Can you work these out from the model? Positions are in its coordinate system, mm. A direction names the side the tool comes from. Round coordinates to 2 decimals unless told otherwise and drop trailing zeros. Loops run counter-clockwise (first coordinate to the right, second up) from the corner with the lowest first, then second, coordinate; pieces in that order, holes last.
(1) Which directions (+Z, -Z, +X, -X, +Y, -Y) give clear straight access to the entire face, cutting with the end or side of a thin tool? Please do faces 1 (the face through (-228.3, -4, 45)), 2 (the face through (-3, -6, 88)), 3 (the face through (228.3, -4, 45)).
(2) I want a section at A-A on y = -3. Write out the boundary of the cut face in (x, z), plus the area to 3 significant figures.
(3) If I drill on line 1 along Z through (x, y) = (-195.5, -5.75); line 2 along X through (y, z) = (-2.5, 55); line 3 along Y through (x, z) = (-77.5, 7), over which ranges is the centre line in solid material (lowest first)?
(4) Will these pins go through, and if not, where does the flat tip stop? pin 1 Ø1.2 at (x, z) = (-230, 41) entering from +Y; pin 2 Ø3 at (x, z) = (70, 9.5) entering from +Y; pin 3 Ø5 at (y, z) = (-5, 43) entering from +X.
(5) I want a section at B-B on x = 31.5. Write out the boundary of the cut face in (y, z).
from build123d import *

# Parameters (mm, degrees)
SKETCH059_W             = 464.6
SKETCH059_H             = 88
PAD022_DEPTH            = 12
SKETCH060_W             = 4
SKETCH060_H             = 88
POCKET036_DEPTH         = 8
SKETCH061_W             = 456.6
SKETCH061_H             = 6
POCKET037_DEPTH         = 6
BODY021_PLACEMENT_ANGLE = 90


with BuildPart() as part:
    # Sketch059 → Pad022 (new body)
    with BuildSketch(Plane.XY):
        with Locations((0, 44)):
            Rectangle(SKETCH059_W, SKETCH059_H)
    extrude(amount=PAD022_DEPTH)

    # Sketch060 (on Face5 of Pad022) → Pocket036 (cut)
    with BuildSketch(Plane(origin=(0, 0, 0), x_dir=(1, 0, 0), z_dir=(0, 0, -1))):
        with Locations((-230.3, -44)):
            Rectangle(SKETCH060_W, SKETCH060_H)
    pocket036 = extrude(amount=-POCKET036_DEPTH, mode=Mode.SUBTRACT)

    # Mirrored013: Pocket036 across Sketch060 V_Axis
    add(pocket036.mirror(Plane(origin=(0, 0, 0), x_dir=(0, 0, -1), z_dir=(1, 0, 0))), mode=Mode.SUBTRACT)

    # Sketch061 (on Face3 of Mirrored013) → Pocket037 (cut)
    with BuildSketch(Plane(origin=(0, 0, 0), x_dir=(1, 0, 0), z_dir=(0, 0, -1))):
        with Locations((0, -9)):
            Rectangle(SKETCH061_W, SKETCH061_H)
    extrude(amount=-POCKET037_DEPTH, mode=Mode.SUBTRACT)


with BuildPart() as part_1:
    # Body021 placement: moved
    add(part.part.rotate(Axis((0, 0, 0), (1, 0, 0)), BODY021_PLACEMENT_ANGLE))


solid = part_1.part
Filled sheet:
1. face 1: +Z, -Z, -X, +Y
1. face 2: +Z, +X, -X, +Y, -Y
1. face 3: +Z, -Z, +X, +Y
2. outline: (-228.3, 0) - (228.3, 0) - (228.3, 6) - (-228.3, 6) - close; (-228.3, 12) - (228.3, 12) - (228.3, 88) - (-228.3, 88) - close
2. area: 37,400 mm2
3. line 1: z = 0 to 6, 12 to 88
3. line 2: x = -228.3 to 228.3
3. line 3: y = -12 to -6
4. pin 1: stops at y = -8
4. pin 2: stops at y = -6
4. pin 3: stops at x = 228.3
5. outline: (-12, 0) - (0, 0) - (0, 6) - (-6, 6) - (-6, 12) - (0, 12) - (0, 88) - (-12, 88) - close
